Verification items for this drawing (mm, ordinates from the low corner). A direction names the side the tool comes from. Round coordinates to 2 decimals unless told otherwise and drop trailing zeros. Loops run counter-clockwise (first coordinate to the right, second up) from the corner with the lowest first, then second, coordinate; pieces in that order, holes last. Notation, with made-up numbers: (-26, 51) - (-21, 51) arc R26 cw to (-21, 82) - close; hole circle Ø2 at (60, 57). An arc over 180 degrees is marked (long way). Answer in a Markdown table with one row per item. Add a question column.
(1) Cross-section at D-D on y = 9. Enter the section's corners in (x, z), then the cut area to 3 significant figures.
(2) Cross-section at C-C on x = 25. Enter the section's corners in (y, z), then the cut area to 3 significant figures.
(3) Cross-section at B-B on z = 2. Enter the section's corners in (x, y).
(4) Cross-section at A-A on y = 55. Enter the section's corners in (x, z).
(5) Gauge pin test, flat ends, axial feed: pin 1 (5 mm diameter, centred on x = 25, y = 55, fed in from -Z); pin 2 (3 mm diameter, centred on y = 7, z = 3, fed in from -X); pin 3 (1 mm diameter, centred on x = 4, z = 4.5, fed in from -Y). Record the tip position at first contact, or that the pin passes through.
(6) Access from +Z, -Z, +X, -X, +Y, -Y to the whole of each face (thin tool, end or side, straight path). Record for the marked faces 1 and 2.
(7) Thickness scan on line 1 along Y through (x, z) = (25, 4.75); line 2 along Y through (x, z) = (24.5, 4); line 3 along Y through (x, z) = (9.75, 4). Record the ranges inside material, lowest first.
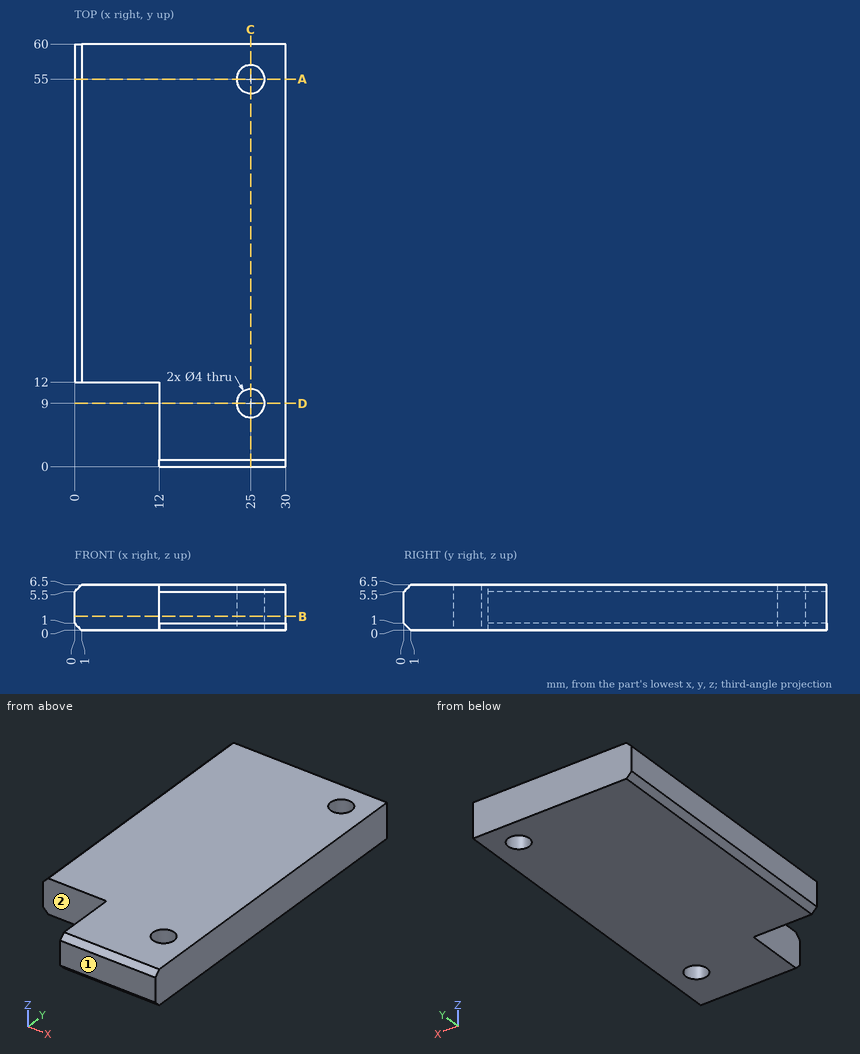
Answers:
| question | item | result |
|---|---|---|
| 1 | outline | (12, 0) - (23, 0) - (23, 6.5) - (12, 6.5) - close; (27, 0) - (30, 0) - (30, 6.5) - (27, 6.5) - close |
| 1 | area | 91.0 mm^2 |
| 2 | outline | (0, 1) - (1, 0) - (7, 0) - (7, 6.5) - (1, 6.5) - (0, 5.5) - close; (11, 0) - (53, 0) - (53, 6.5) - (11, 6.5) - close; (57, 0) - (60, 0) - (60, 6.5) - (57, 6.5) - close |
| 2 | area | 337 mm^2 |
| 3 | outline | (0, 12) - (12, 12) - (12, 0) - (30, 0) - (30, 60) - (0, 60) - close; hole circle Ø4 at (25, 9); hole circle Ø4 at (25, 55) |
| 4 | outline | (0, 1) - (1, 0) - (23, 0) - (23, 6.5) - (1, 6.5) - (0, 5.5) - close; (27, 0) - (30, 0) - (30, 6.5) - (27, 6.5) - close |
| 5 | pin 1 | stops at z = 0 |
| 5 | pin 2 | stops at x = 12 |
| 5 | pin 3 | stops at y = 12 |
| 6 | face 1 | +Z, -Z, +X, -X, -Y |
| 6 | face 2 | +Z, -Z, -X, -Y |
| 7 | line 1 | y = 0 to 7, 11 to 53, 57 to 60 |
| 7 | line 2 | y = 0 to 7.06, 10.94 to 53.06, 56.94 to 60 |
| 7 | line 3 | y = 12 to 60 |
